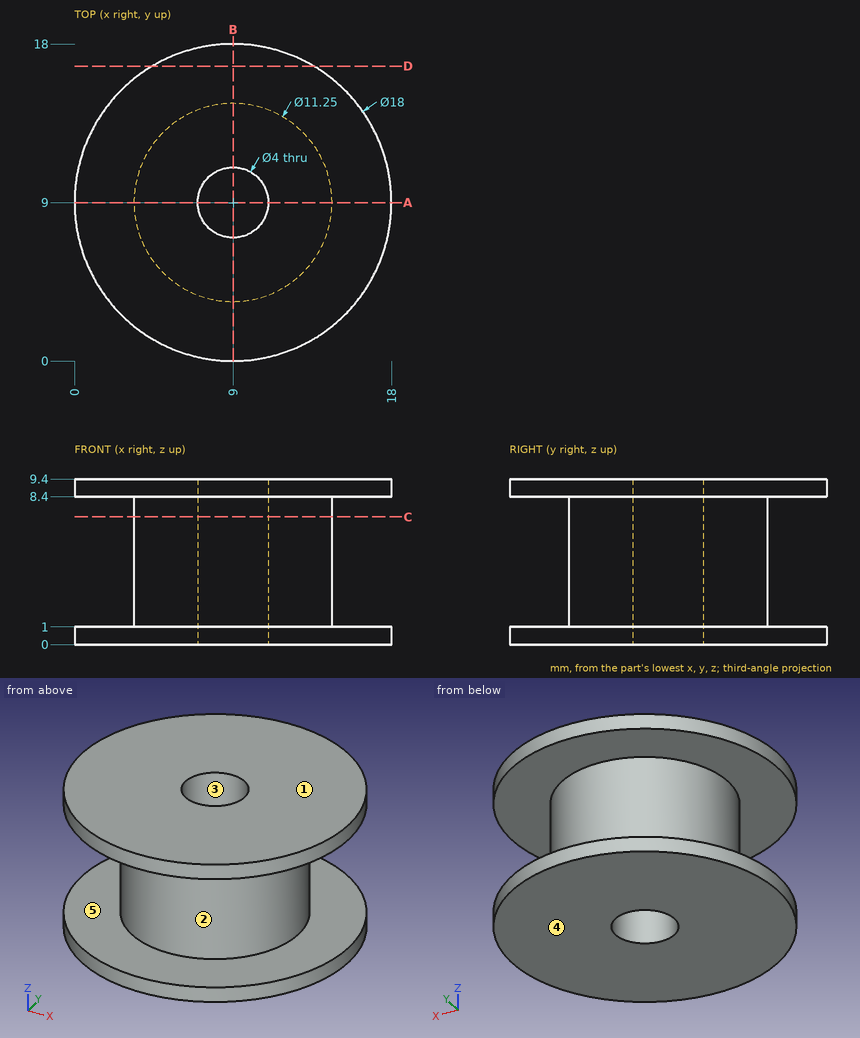
Design review of the part shown in the three views and the two pictorial views. Dimensions are in mm from the part's minimum x, y and z. A direction names the side the tool comes from. Round coordinates to 2 decimals unless told otherwise and drop trailing zeros. Order: outer loops, then holes, each group sorted by start corner. A loop starts at its lowest first (then second) coordinate and runs counter-clockwise, first axis right, second up. Notation, with made-up numbers: (-27.5, 36.5) -> (-3.5, 36.5) arc R16 cw to (-3.5, 51.5) -> close; hole circle Ø5 at (-23.75, 41). An arc over 180 degrees is marked (long way). Write item = value, one per line. Start each with the question number.
1) The part is to be moulded in two halves that separate along Y. For the marked faces 1, 2 and 3, say which applies: +Y half, -Y half, draft (parallel to the pull), parting line (faces both ways), or undercut.
2) Insertion check: pin 1 (2 mm diameter, centred on y = 8.5, z = 3.5, fed in from -X) (3 decimals); pin 2 (1.5 mm diameter, centred on y = 6, z = 6.5, fed in from -X); pin 3 (4 mm diameter, centred on x = 6.5, z = 4, fed in from +Y); pin 4 (3 mm diameter, centred on x = 7.5, y = 8, fed in from +Z). Each pin has a flat end and moves straight along its axis. Give the tip position at first contact, or say it passes through.
3) Tool access review of the marked faces 4 and 5: name each direction out of +Z, -Z, +X, -X, +Y, -Y from which nothing blocks a thin tool from reaching the whole face with its end or side.
4) To check wall thickness, follow line 1 (Z direction, x = 2, y = 12.75); line 2 (Y direction, x = 9, z = 5.5) (3 decimals); line 3 (X direction, y = 8.25, z = 1.75). State the ranges of each line that lie inside material, in increasing order. Write a range as from..to.
5) Take a section at C-C on z = 7.25. State the section outline as (x, y) points (3 decimals).
6) Take a section at D-D on y = 16.75. State the section outline as (x, z) points.
7) Take a section at A-A on y = 9. State the section outline as (x, z) points (3 decimals).
Verdict:
q1.face_1 = draft
q1.face_2 = parting line
q1.face_3 = undercut
q2.pin_1 = 3.375
q2.pin_2 = 3.84
q2.pin_3 = 14.6
q2.pin_4 = 9.4
q3.face_4 = -Z, +X, -X, +Y, -Y
q3.face_5 = none
q4.line_1 = 0..1, 8.4..9.4
q4.line_2 = 3.375..7, 11..14.625
q4.line_3 = 3.43..7.15, 10.85..14.57
q5.outline = circle Ø11.25 at (9, 9); hole circle Ø4 at (9, 9)
q6.outline = (4.42, 0) -> (13.58, 0) -> (13.58, 1) -> (4.42, 1) -> close; (4.42, 8.4) -> (13.58, 8.4) -> (13.58, 9.4) -> (4.42, 9.4) -> close
q7.outline = (0, 0) -> (7, 0) -> (7, 9.4) -> (0, 9.4) -> (0, 8.4) -> (3.375, 8.4) -> (3.375, 1) -> (0, 1) -> close; (11, 0) -> (18, 0) -> (18, 1) -> (14.625, 1) -> (14.625, 8.4) -> (18, 8.4) -> (18, 9.4) -> (11, 9.4) -> close
